The listing builds one solid part. Answer for the finished solid, in the listing's coordinates (mm). A direction names the side the tool comes from. Give positions to 0.01 mm unless a question says otherwise; leave off trailing zeros. Answer as CSV lines item,"result". Start each with the question number.
1) Flat-ended cylindrical pins translate along their axes: pin 1 (1.5 mm diameter, centred on x = 7.5, y = 6.5, fed in from +Z); pin 2 (2 mm diameter, centred on x = -3, z = 2.5, fed in from +Y); pin 3 (2 mm diameter, centred on y = -6.5, z = 3, fed in from +X); pin 4 (1.5 mm diameter, centred on x = -0.5, z = 2.5, fed in from +Y). Find the tip coordinate at first contact, or state that the pin passes through.
2) Find the intervals of material crossed by line 1 along Y through (x, z) = (0, 7.5) (3 decimals); line 2 along X through (y, z) = (-8.5, 3.75); line 3 along X through (y, z) = (9, 3.75), in increasing order.
3) For faces 1 (the face through (9.434, -2.196, 4.696)), 2 (the face through (-8.92, -3.77, 4.7)), 3 (the face through (-3.17, -9.15, 4.7)), 4 (the face through (-8.77, 4.11, 4.7)), 5 (the face through (-0.933, 9.607, 4.696)), determine the directions among +Z, -Z, +X, -X, +Y, -Y from which every point of the face is accessible in a straight line to the end or side of a thin tool.
```python
from build123d import *

# Parameters (mm, degrees)
SKETCH3_R         = 10.795
GEARBODY_DEPTH    = 9.525
TOOTHCUT_DEPTH    = 10.525
CIRPATTERN1_COUNT = 15
BOREDIA_R         = 3.96875
BORE_DEPTH        = 12700


with BuildPart() as part:
    # Sketch3 → gearBody (new body)
    with BuildSketch(Plane.XY):
        Circle(SKETCH3_R)
    extrude(amount=GEARBODY_DEPTH)

    # Sketch2 → toothCut (cut, through all)
    with BuildSketch(Plane.XY):
        with BuildLine():
            ThreePointArc((7.864672513, -1.163016041), (7.895149368, -0.933968145), (7.918956949, -0.704131297))
            ThreePointArc((7.918956949, -0.704131297), (8.083653363, -0.376064465), (8.4281848, -0.249372536))
            ThreePointArc((8.4281848, -0.249372536), (10.244786828, 0.166211992), (11.641974978, 1.399345683))
            ThreePointArc((11.641974978, 1.399345683), (11.644578548, -1.377512307), (10.99412895, -4.077116426))
            ThreePointArc((10.99412895, -4.077116426), (9.923230012, -2.552016793), (8.253736923, -1.724039588))
            ThreePointArc((8.253736923, -1.724039588), (7.948275924, -1.520455861), (7.864672513, -1.163016041))
        make_face()
    toothcut = extrude(amount=TOOTHCUT_DEPTH, mode=Mode.SUBTRACT)

    # CirPattern1: toothCut ×15 about axis
    cirpattern1_axis = Axis((0, 0, 0), (0, 0, 1))
    for i in range(1, CIRPATTERN1_COUNT):
        add(toothcut.rotate(cirpattern1_axis, i * 360 / CIRPATTERN1_COUNT), mode=Mode.SUBTRACT)

    # boreDia → bore (cut, symmetric)
    with BuildSketch(Plane.XY):
        Circle(BOREDIA_R)
    extrude(amount=BORE_DEPTH, both=True, mode=Mode.SUBTRACT)


solid = part.part
```
Ans:
1,pin 1,"through"
1,pin 2,"y = 10.61"
1,pin 3,"x = 8.25"
1,pin 4,"y = 10.19"
2,line 1,"-10.795 to -3.969, 3.969 to 7.95"
2,line 2,"-4.93 to -2.77, -1.14 to 0.92, 2.51 to 4.68"
2,line 3,"-5.96 to -5.64, -2.81 to -0.73, 0.97 to 3.05"
3,face 1,"+Z, -Z, +X"
3,face 2,"+Z, -Z"
3,face 3,"+Z, -Z, -Y"
3,face 4,"+Z, -Z, -X"
3,face 5,"+Z, -Z, +Y"
